```python
from build123d import *

# Parameters (mm, degrees)
ESQUISSE1_W             = 206
ESQUISSE1_H             = 278.55339059
BOSS_EXTRU_1_DEPTH      = 4
ESQUISSE2_W             = 216
ESQUISSE2_H             = 290.55339059
BOSS_EXTRU_2_DEPTH      = 4
ESQUISSE3_W             = 156
ESQUISSE3_H             = 248.55339059
ENL_V_MAT_EXTRU_1_DEPTH = 8
ENL_V_MAT_EXTRU_2_DEPTH = 2
ESQUISSE5_R             = 1.5
ENL_V_MAT_EXTRU_3_DEPTH = 4
ESQUISSE6_R             = 3
ENL_V_MAT_EXTRU_4_DEPTH = 4
ESQUISSE7_R             = 1
ENL_V_MAT_EXTRU_5_DEPTH = 739.46020643


with BuildPart() as part:
    # Esquisse1 → Boss.-Extru.1 (new body)
    with BuildSketch(Plane.XY):
        with Locations((121.349909903, 555.619376292)):
            Rectangle(ESQUISSE1_W, ESQUISSE1_H)
    extrude(amount=BOSS_EXTRU_1_DEPTH)

    # Esquisse2 → Boss.-Extru.2 (add)
    with BuildSketch(Plane.XY.offset(4)):
        with Locations((121.349909903, 556.619376292)):
            Rectangle(ESQUISSE2_W, ESQUISSE2_H)
    extrude(amount=BOSS_EXTRU_2_DEPTH)

    # Esquisse3 → Enlèv. mat.-Extru.1 (cut)
    with BuildSketch(Plane(origin=(0, 0, 0), x_dir=(-1, 0, 0), z_dir=(0, 0, -1))):
        with Locations((-131.349909903, 555.619376292)):
            Rectangle(ESQUISSE3_W, ESQUISSE3_H)
    extrude(amount=-ENL_V_MAT_EXTRU_1_DEPTH, mode=Mode.SUBTRACT)

    # Esquisse4 → Enlèv. mat.-Extru.2 (cut)
    with BuildSketch(Plane(origin=(0, 0, 0), x_dir=(-1, 0, 0), z_dir=(0, 0, -1))):
        with BuildLine():
            Line((-212.228589559, 684.896071587), (-50.471230246, 684.896071587))
            ThreePointArc((-50.471230246, 684.896071587), (-48.349909903, 684.896071587), (-48.349909903, 682.774751243))
            Line((-48.349909903, 682.774751243), (-48.349909903, 428.418245014))
            ThreePointArc((-48.349909903, 428.418245014), (-48.51477084, 426.464915653), (-50.471230246, 426.342680997))
            Line((-50.471230246, 426.342680997), (-51.11665592, 426.342680997))
            Line((-51.11665592, 426.342680997), (-211.583163885, 426.342680997))
            Line((-211.583163885, 426.342680997), (-212.228589559, 426.342680997))
            ThreePointArc((-212.228589559, 426.342680997), (-214.185048965, 426.464915653), (-214.349909903, 428.418245014))
            Line((-214.349909903, 428.418245014), (-214.349909903, 682.774751243))
            ThreePointArc((-214.349909903, 682.774751243), (-214.349909903, 684.896071587), (-212.228589559, 684.896071587))
        make_face()
    extrude(amount=-ENL_V_MAT_EXTRU_2_DEPTH, mode=Mode.SUBTRACT)

    # Esquisse5 → Enlèv. mat.-Extru.3 (cut)
    with BuildSketch(Plane(origin=(0, 0, 4), x_dir=(-1, 0, 0), z_dir=(0, 0, -1))):
        with Locations((-219.349909903, 696.896071587)):
            Circle(ESQUISSE5_R)
        with Locations(Location((-24.067400597, 696.896071587, 0), (0, 0, 180))):
            Circle(ESQUISSE5_R)
    extrude(amount=-ENL_V_MAT_EXTRU_3_DEPTH, mode=Mode.SUBTRACT)

    # Esquisse6 → Enlèv. mat.-Extru.4 (cut)
    with BuildSketch(Plane(origin=(0, 0, 0), x_dir=(-1, 0, 0), z_dir=(0, 0, -1))):
        with Locations((-24.067400597, 696.896071587)):
            Circle(ESQUISSE6_R)
        with Locations((-219.349909903, 696.896071587)):
            Circle(ESQUISSE6_R)
    extrude(amount=-ENL_V_MAT_EXTRU_4_DEPTH, mode=Mode.SUBTRACT)

    # Esquisse7 → Enlèv. mat.-Extru.5 (cut, through all)
    with BuildSketch(Plane.XY.offset(8)):
        with Locations((49.662982919, 421.342680997)):
            Circle(ESQUISSE7_R)
        with Locations((194.662982919, 421.342680997)):
            Circle(ESQUISSE7_R)
    extrude(amount=-ENL_V_MAT_EXTRU_5_DEPTH, mode=Mode.SUBTRACT)


solid = part.part
```
Design review of the part built by this model. Coordinates are the model's own, in mm. A direction names the side the tool comes from. Round coordinates to 2 decimals unless told otherwise and drop trailing zeros. Write each loop counter-clockwise with the first axis right and the second up, starting at its lowest first coordinate (ties: lowest second). Pieces come first, ordered by that corner, then holes.
Item 1: For probe 1 along Y at (x, z) = (194.5, 0.75); probe 2 along X at (y, z) = (437.5, 3); probe 3 along Y at (x, z) = (100.5, 1), list the stretches that pass through material, from the lowest coordinate up.
Item 2: We need section A-A on x = 142.5. Write out the cut boundary in (y, z), and give its area (3 significant figures).
Item 3: The part is to be moulded in two halves that separate along X. For faces 1 (the flat face through (209.35, 554, 5)), 2 (the flat face through (48, 559, 8)), 3 (the flat face through (132, 431.343, 5)), say which applies: +X half, -X half, draft (parallel to the pull), parting line (faces both ways), or undercut.
Item 4: Clearance check with flat-ended pins moving along their axes: pin 1 Ø0.6 at (y, z) = (588, 1.5) entering from +X; pin 2 Ø1 at (x, z) = (20, 2.5) entering from +Y; pin 3 Ø3 at (x, z) = (143.5, 2) entering from -Y. State where each tip first meets the part, or that it passes through.
Item 5: We need section B-B on y = 619.5. Write out the cut boundary in (x, z).
Item 6: For faces 4 (the flat face through (53.35, 554, 5)), 5 (the flat face through (45, 515, 0)), 6 (the flat face through (51, 595, 2)), list the 3-axis set-ups (+Z, -Z, +X, -X, +Y, -Y) from which the entire face can be reached by the end or side of a thin tool; tool diameter is ignored.
Returned:
1. probe 1: y = 416.34 to 420.36, 422.33 to 426.34, 684.9 to 694.9
1. probe 2: x = 18.35 to 53.35, 209.35 to 224.35
1. probe 3: y = 416.34 to 426.34, 684.9 to 694.9
2. outline: (411.34, 4) - (416.34, 4) - (416.34, 0) - (426.34, 0) - (426.34, 2) - (431.34, 2) - (431.34, 8) - (411.34, 8) - close; (679.9, 2) - (684.9, 2) - (684.9, 0) - (694.9, 0) - (694.9, 4) - (701.9, 4) - (701.9, 8) - (679.9, 8) - close
2. area: 268 mm2
3. face 1: undercut
3. face 2: draft
3. face 3: undercut
4. pin 1: stops at x = 224.35
4. pin 2: stops at y = 694.9
4. pin 3: stops at y = 416.34
5. outline: (13.35, 4) - (18.35, 4) - (18.35, 0) - (48.35, 0) - (48.35, 2) - (53.35, 2) - (53.35, 8) - (13.35, 8) - close; (209.35, 2) - (214.35, 2) - (214.35, 0) - (224.35, 0) - (224.35, 4) - (229.35, 4) - (229.35, 8) - (209.35, 8) - close
6. face 4: +Z, -Z
6. face 5: -Z, +X, -X, +Y, -Y
6. face 6: -Z
